For this review, take the finished solid that the model builds, in its own axes (mm). Coordinates: 2 decimals unless noted, no trailing zeros. Loops run counter-clockwise (first coordinate to the right, second up) from the corner with the lowest first, then second, coordinate; pieces in that order, holes last. Notation, with made-up numbers: (77, 9.5) -> (101, 9.5) arc R12 cw to (101, 19.5) -> close; hole circle Ø4 at (54, 83.5). An arc over 180 degrees is marked (long way). Use a Markdown table: item, result.
from build123d import *

# Parameters (mm, degrees)
SKETCH1_W           = 142.494
SKETCH1_H           = 75.692
BOSS_EXTRUDE2_DEPTH = 6.35
FILLET4_R           = 12.7


with BuildPart() as part:
    # Sketch1 → Boss-Extrude2 (new body)
    with BuildSketch(Plane(origin=(0, 0, 0), x_dir=(1, 0, 0), z_dir=(0, 1, 0))):
        Polygon((-71.247, 37.846), (0, 37.846), (0, 215.646), align=None)
        Polygon((0, 215.646), (0, 37.846), (71.247, 37.846), align=None)
        Rectangle(SKETCH1_W, SKETCH1_H)
    extrude(amount=BOSS_EXTRUDE2_DEPTH)

    # Fillet4
    fillet4_edges = [part.edges().sort_by_distance(p)[0] for p in [
        (0, 3.175, -215.646),
    ]]
    fillet(fillet4_edges, radius=FILLET4_R)


solid = part.part
(1) Take a section at A-A on y = 5. Write out the cut boundary in (x, z), plus the area to 3 significant figures.
Found:
| item | result |
|---|---|
| outline | (-71.25, -37.85) -> (-11.79, -186.23) arc R12.7 ccw to (11.79, -186.23) -> (71.25, -37.85) -> (71.25, 37.85) -> (-71.25, 37.85) -> close |
| area | 23,200 mm^2 |
(2) For pin 1 Ø3 at (y, z) = (1, -109) entering from -X, flat-tipped, find the tip position at first contact; note if it passes through.
Found:
| item | result |
|---|---|
| pin 1 | stops at x = -43.34 |
(3) For line 1 along Z through (x, y) = (-1, 2.75); line 2 along X through (y, z) = (4, -157); line 3 along Z through (x, y) = (-63, 2.5), list the stretches that pass through material, from the lowest coordinate up.
Found:
| item | result |
|---|---|
| line 1 | z = -194.16 to 37.85 |
| line 2 | x = -23.5 to 23.5 |
| line 3 | z = -58.43 to 37.85 |
(4) Take a section at B-B on x = -48.5. Write out the cut boundary in (y, z), plus the area to 3 significant figures.
Found:
| item | result |
|---|---|
| outline | (0, -94.61) -> (6.35, -94.61) -> (6.35, 37.85) -> (0, 37.85) -> close |
| area | 841 mm^2 |
(5) Take a section at C-C on z = -178.5. Write out the cut boundary in (x, y), plus the area to 3 significant figures.
Found:
| item | result |
|---|---|
| outline | (-14.88, 0) -> (14.88, 0) -> (14.88, 6.35) -> (-14.88, 6.35) -> close |
| area | 189 mm^2 |
